Here's how the part is built. I have some questions about the finished solid (model axes, mm). Face numbers are marked on the shaded views. A direction names the side the tool comes from. Give positions to 0.01 mm unless a question says otherwise; leave off trailing zeros. Order: outer loops, then holes, each group sorted by start corner. A loop starts at its lowest first (then second) coordinate and runs counter-clockwise, first axis right, second up.
from build123d import *

# Parameters (mm, degrees)
F0_W     = 84
F0_H     = 40
F0_R     = 1.45
F1_DEPTH = 1
F2_DEPTH = 7.6
F3_W     = 82
F3_H     = 38
F3_W_2   = 80.5
F3_H_2   = 36.5
F4_DEPTH = 1
F5_W     = 68
F5_H     = 20
F6_DEPTH = 5
F7_W     = 11
F7_H     = 13.6534924152
F8_DEPTH = 1.75
F9_SIZE  = 1


with BuildPart() as f1:
    # F0 (on Top) → F1 (new body)
    with BuildSketch(Plane.XY):
        with Locations((-0.3290896534, 0.19)):
            Rectangle(F0_W, F0_H)
        Polygon((-40.5790896534, 13.39), (-40.5790896534, 18.44), (-35.5290896534, 18.44), (34.8709103466, 18.44), (39.9209103466, 18.44), (39.9209103466, 13.39), (39.9209103466, -13.01), (39.9209103466, -18.06), (34.8709103466, -18.06), (-35.5290896534, -18.06), (-40.5790896534, -18.06), (-40.5790896534, -13.01), align=None, mode=Mode.SUBTRACT)
        with BuildLine():
            Line((34.8709103466, 18.44), (-35.5290896534, 18.44))
            Line((-35.5290896534, 18.44), (-35.5290896534, 15.89))
            ThreePointArc((-35.5290896534, 15.89), (-36.2613227005, 14.122233047), (-38.0290896534, 13.39))
            Line((-38.0290896534, 13.39), (-40.5790896534, 13.39))
            Line((-40.5790896534, 13.39), (-40.5790896534, -13.01))
            Line((-40.5790896534, -13.01), (-38.0290896534, -13.01))
            ThreePointArc((-38.0290896534, -13.01), (-36.2613227005, -13.742233047), (-35.5290896534, -15.51))
            Line((-35.5290896534, -15.51), (-35.5290896534, -18.06))
            Line((-35.5290896534, -18.06), (34.8709103466, -18.06))
            Line((34.8709103466, -18.06), (34.8709103466, -15.51))
            ThreePointArc((34.8709103466, -15.51), (35.6031433936, -13.742233047), (37.3709103466, -13.01))
            Line((37.3709103466, -13.01), (39.9209103466, -13.01))
            Line((39.9209103466, -13.01), (39.9209103466, 13.39))
            Line((39.9209103466, 13.39), (37.3709103466, 13.39))
            ThreePointArc((37.3709103466, 13.39), (35.6031433936, 14.122233047), (34.8709103466, 15.89))
            Line((34.8709103466, 15.89), (34.8709103466, 18.44))
        make_face()
        with BuildLine():
            Line((-35.5290896534, 18.44), (-40.5790896534, 18.44))
            Line((-40.5790896534, 18.44), (-40.5790896534, 13.39))
            Line((-40.5790896534, 13.39), (-38.0290896534, 13.39))
            ThreePointArc((-38.0290896534, 13.39), (-36.2613227005, 14.122233047), (-35.5290896534, 15.89))
            Line((-35.5290896534, 15.89), (-35.5290896534, 18.44))
        make_face()
        with Locations((-38.0290896534, 15.89)):
            Circle(F0_R, mode=Mode.SUBTRACT)
        with BuildLine():
            Line((39.9209103466, 18.44), (34.8709103466, 18.44))
            Line((34.8709103466, 18.44), (34.8709103466, 15.89))
            ThreePointArc((34.8709103466, 15.89), (35.6031433936, 14.122233047), (37.3709103466, 13.39))
            Line((37.3709103466, 13.39), (39.9209103466, 13.39))
            Line((39.9209103466, 13.39), (39.9209103466, 18.44))
        make_face()
        with Locations((37.3709103466, 15.89)):
            Circle(F0_R, mode=Mode.SUBTRACT)
        with BuildLine():
            Line((-38.0290896534, -13.01), (-40.5790896534, -13.01))
            Line((-40.5790896534, -13.01), (-40.5790896534, -18.06))
            Line((-40.5790896534, -18.06), (-35.5290896534, -18.06))
            Line((-35.5290896534, -18.06), (-35.5290896534, -15.51))
            ThreePointArc((-35.5290896534, -15.51), (-36.2613227005, -13.742233047), (-38.0290896534, -13.01))
        make_face()
        with Locations((-38.0290896534, -15.51)):
            Circle(F0_R, mode=Mode.SUBTRACT)
        with BuildLine():
            Line((39.9209103466, -18.06), (39.9209103466, -13.01))
            Line((39.9209103466, -13.01), (37.3709103466, -13.01))
            ThreePointArc((37.3709103466, -13.01), (35.6031433936, -13.742233047), (34.8709103466, -15.51))
            Line((34.8709103466, -15.51), (34.8709103466, -18.06))
            Line((34.8709103466, -18.06), (39.9209103466, -18.06))
        make_face()
        with Locations((37.3709103466, -15.51)):
            Circle(F0_R, mode=Mode.SUBTRACT)
        with Locations((-38.0290896534, 15.89)):
            Circle(F0_R)
        with Locations((-38.0290896534, -15.51)):
            Circle(F0_R)
        with Locations((37.3709103466, 15.89)):
            Circle(F0_R)
        with Locations((37.3709103466, -15.51)):
            Circle(F0_R)
    extrude(amount=F1_DEPTH)

    # F0 (on Top) → F2 (join)
    with BuildSketch(Plane.XY):
        with Locations((-0.3290896534, 0.19)):
            Rectangle(F0_W, F0_H)
        Polygon((-40.5790896534, 13.39), (-40.5790896534, 18.44), (-35.5290896534, 18.44), (34.8709103466, 18.44), (39.9209103466, 18.44), (39.9209103466, 13.39), (39.9209103466, -13.01), (39.9209103466, -18.06), (34.8709103466, -18.06), (-35.5290896534, -18.06), (-40.5790896534, -18.06), (-40.5790896534, -13.01), align=None, mode=Mode.SUBTRACT)
    extrude(amount=F2_DEPTH)

    # F3 (on face) → F4 (join)
    with BuildSketch(Plane.XY.offset(7.6)):
        with Locations((-0.3290896534, 0.19)):
            Rectangle(F3_W, F3_H)
        with Locations((-0.3290896534, 0.19)):
            Rectangle(F3_W_2, F3_H_2, mode=Mode.SUBTRACT)
    extrude(amount=F4_DEPTH)

    # F5 (on face) → F6 (cut)
    with BuildSketch(Plane.XY):
        with Locations((-0.3290896534, 0.19)):
            Rectangle(F5_W, F5_H)
    extrude(amount=F6_DEPTH, mode=Mode.SUBTRACT)

    # F7 (on face) → F8 (join)
    with BuildSketch(Plane.YZ.offset(41.6709103466)):
        with Locations((7.94, 9.7732537924)):
            Rectangle(F7_W, F7_H)
    extrude(amount=-F8_DEPTH)

    # F9
    f9_edges = [f1.edges().sort_by_distance(p)[0] for p in [
        (-0.32909, -19.81, 0),
        (41.67091, 0.19, 0),
        (-0.32909, 20.19, 0),
        (-42.32909, 0.19, 0),
    ]]
    chamfer(f9_edges, length=F9_SIZE)


solid = f1.part
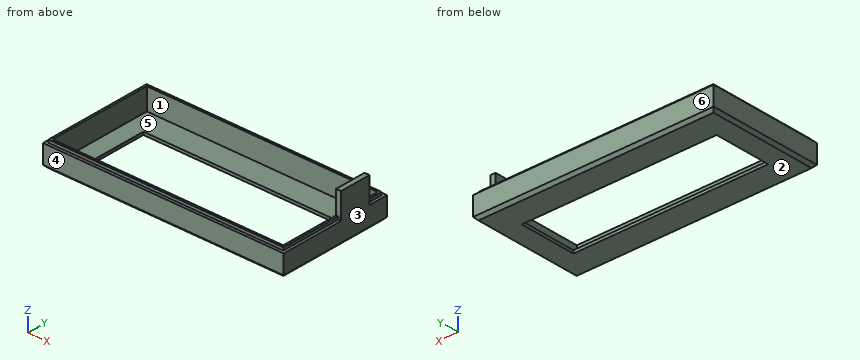
Q1. If we section it at D-D on y = -4.5: List the corners of the cut face in (x, z) for me, plus the area to 3 significant figures.
Filled sheet:
outline: (-42.33, 1) - (-41.33, 0) - (-34.33, 0) - (-34.33, 1) - (-40.58, 1) - (-40.58, 8.6) - (-41.33, 8.6) - (-41.33, 7.6) - (-42.33, 7.6) - close; (33.67, 0) - (40.67, 0) - (41.67, 1) - (41.67, 7.6) - (40.67, 7.6) - (40.67, 8.6) - (39.92, 8.6) - (39.92, 1) - (33.67, 1) - close
area: 39.6 mm2
Q2. I need wall thicknesses on L1, parallel to X at y = -4, z = 1.5; L2, parallel to X at y = 6.5, z = 8.5; L3, parallel to Y at x = -30, z = 7.25. Which ranges of each line are inside material? Lowest first, please.
Filled sheet:
L1: x = -42.33 to -40.58, 39.92 to 41.67
L2: x = -41.33 to -40.58, 39.92 to 41.67
L3: y = -19.81 to -18.06, 18.44 to 20.19
Q3. If we section it at C-C on z = 5.75: List the corners of the cut face in (x, y) for me.
Filled sheet:
outline: (-42.33, -19.81) - (41.67, -19.81) - (41.67, 20.19) - (-42.33, 20.19) - close; hole (-40.58, -18.06) - (39.92, -18.06) - (39.92, 18.44) - (-40.58, 18.44) - close
Q4. If we section it at A-A on y = 5: List the corners of the cut face in (x, z) for me, plus the area to 3 significant figures.
Filled sheet:
outline: (-42.33, 1) - (-41.33, 0) - (-34.33, 0) - (-34.33, 1) - (-40.58, 1) - (-40.58, 8.6) - (-41.33, 8.6) - (-41.33, 7.6) - (-42.33, 7.6) - close; (33.67, 0) - (40.67, 0) - (41.67, 1) - (41.67, 16.6) - (39.92, 16.6) - (39.92, 1) - (33.67, 1) - close
area: 54.6 mm2
Q5. For the marked faces 1 and 2, which set-ups out of +Z, -Z, +X, -X, +Y, -Y let a thin tool reach every point of the face, with its end or its side?
Filled sheet:
face 1: +Z
face 2: -Z, +X, -X, +Y, -Y
Q6. I'm going to push flat-ended pins straight in: P1, Ø1.4, axis at x = 41, z = 13, coming from the -Y side; P2, Ø1.1, axis at y = 15, z = 8, coming from the +X side; P3, Ø0.5, axis at x = 10, z = 0.5, coming from the +Y side; P4, Ø6, axis at x = -13.5, y = 7, coming from the +Z side. Where does each tip first touch, or does it pass through?
Filled sheet:
P1: stops at y = 2.44
P2: stops at x = 41.67
P3: stops at y = 19.94
P4: passes through
Q7. If we section it at B-B on x = -17: List the corners of the cut face in (y, z) for me.
Filled sheet:
outline: (-19.81, 1) - (-18.81, 0) - (-9.81, 0) - (-9.81, 1) - (-18.06, 1) - (-18.06, 8.6) - (-18.81, 8.6) - (-18.81, 7.6) - (-19.81, 7.6) - close; (10.19, 0) - (19.19, 0) - (20.19, 1) - (20.19, 7.6) - (19.19, 7.6) - (19.19, 8.6) - (18.44, 8.6) - (18.44, 1) - (10.19, 1) - close
Q8. Thinking about a two-plate mould opening in Y: for the marked faces 3, 4, 5 and 6, which applies, released by +Y, released by -Y, zero draft, split by the parting line, or undercut?
Filled sheet:
face 3: zero draft
face 4: released by -Y
face 5: undercut
face 6: released by +Y
